```python
from build123d import *

# Parameters (mm, degrees)
SKETCH_1_W          = 74
SKETCH_1_H          = 80
SKETCH_1_R          = 1.45
EXTRUDE_1_DEPTH     = 5
FILLET_1_R          = 6
SKETCH_2_W          = 55
SKETCH_2_H          = 80
CUT_EXTRUDE_1_DEPTH = 2
FILLET_2_R          = 10


with BuildPart() as part:
    # 草图1 → 凸台-拉伸1 (new body)
    with BuildSketch(Plane(origin=(0, 0, 0), x_dir=(1, 0, 0), z_dir=(0, 1, 0))):
        Rectangle(SKETCH_1_W, SKETCH_1_H)
        with Locations(Location((-33, 21, 0), (0, 0, 270))):
            Circle(SKETCH_1_R, mode=Mode.SUBTRACT)
        with Locations(Location((-33, -21, 0), (0, 0, 90))):
            Circle(SKETCH_1_R, mode=Mode.SUBTRACT)
        with Locations(Location((33, -21, 0), (0, 0, 270))):
            Circle(SKETCH_1_R, mode=Mode.SUBTRACT)
        with Locations(Location((33, 21, 0), (0, 0, 90))):
            Circle(SKETCH_1_R, mode=Mode.SUBTRACT)
    extrude(amount=EXTRUDE_1_DEPTH)

    # 圆角1
    fillet_1_edges = [part.edges().sort_by_distance(p)[0] for p in [
        (37, 2.5, 40),
        (-37, 2.5, 40),
        (-37, 2.5, -40),
        (37, 2.5, -40),
    ]]
    fillet(fillet_1_edges, radius=FILLET_1_R)

    # 草图2 → 切除-拉伸1 (cut)
    with BuildSketch(Plane(origin=(0, 5, 0), x_dir=(1, 0, 0), z_dir=(0, 1, 0))):
        Rectangle(SKETCH_2_W, SKETCH_2_H)
    extrude(amount=-CUT_EXTRUDE_1_DEPTH, mode=Mode.SUBTRACT)

    # 圆角2
    # the kernel refuses this fillet: 10 mm, written as the material it adds along each edge
    with BuildSketch(Plane(origin=(-27.5, 3, -40), x_dir=(1, 0, 0), z_dir=(0, 0, 1))) as fillet_2_piece_1:
        with BuildLine():
            CenterArc((6, 10), FILLET_2_R, 233.130102354, 36.869897646)
            Line((0, 2), (-0.12, 1.84))
            ThreePointArc((-0.12, 1.84), (-0.2, 1), (-0.2, 0))
            Line((-0.2, 0), (0, -0.2))
            Line((0, -0.2), (6, -0.2))
            Line((6, -0.2), (6, 0))
        make_face()
    extrude(amount=80)
    with BuildSketch(Plane(origin=(27.5, 3, 40), x_dir=(0, 1, 0), z_dir=(0, 0, -1))) as fillet_2_piece_2:
        with BuildLine():
            CenterArc((10, -6), FILLET_2_R, 143.130102354, 36.869897646)
            Line((0, -6), (-0.2, -6))
            Line((-0.2, -6), (-0.2, 0))
            Line((-0.2, 0), (0, 0.2))
            ThreePointArc((0, 0.2), (1, 0.2), (1.84, 0.12))
            Line((1.84, 0.12), (2, 0))
        make_face()
    extrude(amount=80)


solid = part.part
```
Check sheet for the modelled part. Datum: model origin and axes. Units: mm. A direction names the side the tool comes from. Round coordinates to 2 decimals unless told otherwise and drop trailing zeros. Loops run counter-clockwise (first coordinate to the right, second up) from the corner with the lowest first, then second, coordinate; pieces in that order, holes last. Notation, with made-up numbers: (9, 20) - (68, 20) arc R26 cw to (68, 56) - close; hole circle Ø4 at (-5.5, 0). An arc over 180 degrees is marked (long way). Answer as a JSON object with one key per item and string values. Group by question number.
Q1. Sectioned sample at D-D, the plane x = 14. Enter the section's corners in (y, z), plus the area to 3 significant figures.
Q2. Scan lines: line 1 along X through (y, z) = (2.75, -21); line 2 along Z through (x, y) = (33.5, 0.25); line 3 along X through (y, z) = (3.95, -21). Record each from-to range of solid material in increasing order. Write a range as [from, to].
Q3. Sectioned sample at C-C, the plane z = 3.5. Enter the section's corners in (x, y).
Q4. Set-up check for faces 1 (the face through (0, 2, 40)), 2 (the face through (0, 3, -1)): record each of +Z, -Z, +X, -X, +Y, -Y from which the full face is reachable in a straight line by a thin tool's end or side.
Q5. Mould release check, pull along X, two halves, no side actions. Record for faces 3 (the face through (32.445, 2.465, 22.339)), 4 (the face through (35.196, 2.535, -38.289)), 5 (the face through (-1, 0, -1)): released by +X, released by -X, zero draft, split by the parting line, or undercut.
Q6. Sectioned sample at A-A, the plane z = 21. Enter the section's corners in (x, y), plus the area to 3 significant figures.
Q7. Sectioned sample at B-B, the plane x = 33. Enter the section's corners in (y, z).
Q8. Gauge pin test, flat ends, axial feed: P1, Ø2, axis at x = 22.5, z = 28.5, coming from the +Y side; P2, Ø21.5, axis at x = 9, z = -12.5, coming from the +Y side; P3, Ø4, axis at x = 22, z = 21, coming from the +Y side. Record the tip position at first contact, or that the pin passes through.
Solution:
{
 "1": {"outline": "(0, -40) - (3, -40) - (3, 40) - (0, 40) - close", "area": "240 mm²"},
 "2": {"line 1": "x = [-37, -34.45], [-31.55, 31.55], [34.45, 37]", "line 2": "z = [-39.45, -22.36], [-19.64, 19.64], [22.36, 39.45]", "line 3": "x = [-37, -34.45], [-31.55, -25.75], [25.75, 31.55], [34.45, 37]"},
 "3": {"outline": "(-37, 0) - (37, 0) - (37, 5) - (27.5, 5) arc R10 cw to (21.5, 3) - (-21.5, 3) arc R10 cw to (-27.5, 5) - (-37, 5) - close"},
 "4": {"face 1": "+Z, +X, -X, +Y, -Y", "face 2": "+Z, -Z, +Y"},
 "5": {"face 3": "undercut", "face 4": "released by +X", "face 5": "zero draft"},
 "6": {"outline": "(-37, 0) - (-34.45, 0) - (-34.45, 5) - (-37, 5) - close; (-31.55, 0) - (31.55, 0) - (31.55, 5) - (27.5, 5) arc R10 cw to (21.5, 3) - (-21.5, 3) arc R10 cw to (-27.5, 5) - (-31.55, 5) - close; (34.45, 0) - (37, 0) - (37, 5) - (34.45, 5) - close", "area": "239 mm²"},
 "7": {"outline": "(0, -39.66) - (5, -39.66) - (5, -22.45) - (0, -22.45) - close; (0, -19.55) - (5, -19.55) - (5, 19.55) - (0, 19.55) - close; (0, 22.45) - (5, 22.45) - (5, 39.66) - (0, 39.66) - close"},
 "8": {"P1": "stops at y = 3.2", "P2": "stops at y = 3", "P3": "stops at y = 3.32"}
}
